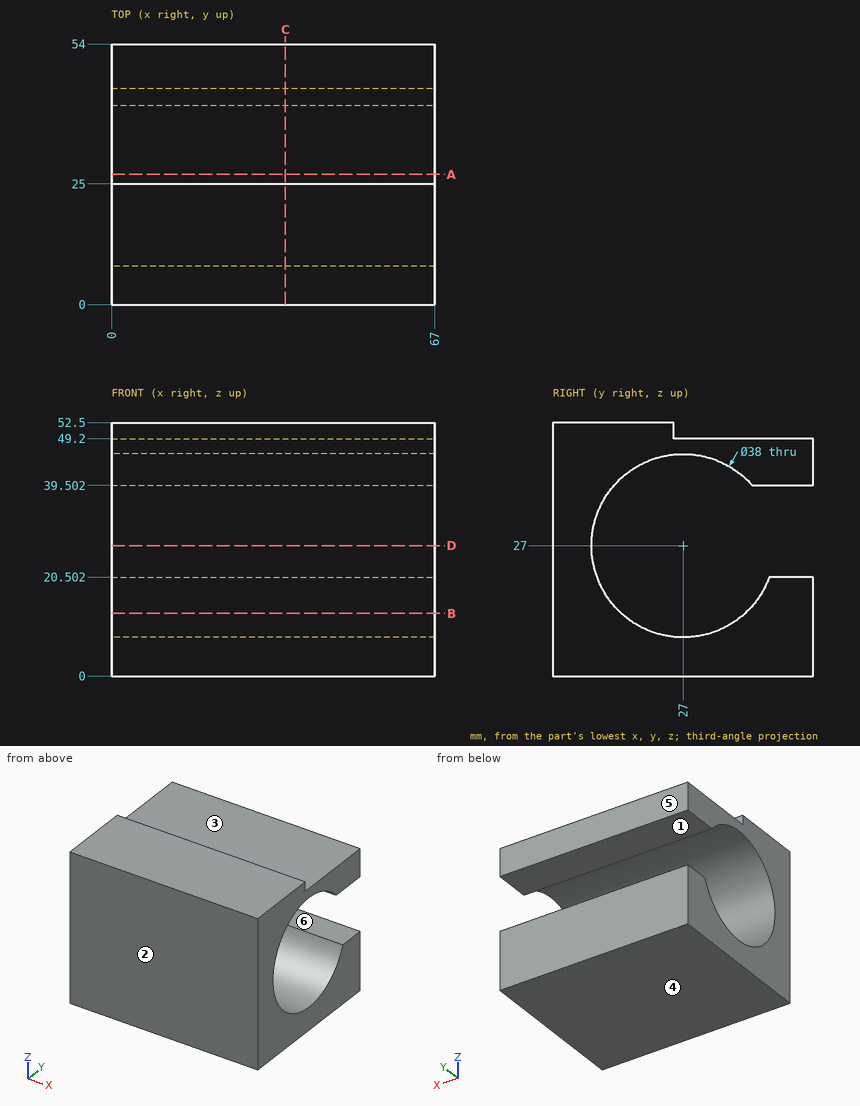
Check sheet for the drawn part. Datum: minimum x, y, z corner. Units: mm. A direction names the side the tool comes from. Round coordinates to 2 decimals unless told otherwise and drop trailing zeros. Order: outer loops, then holes, each group sorted by start corner. A loop starts at its lowest first (then second) coordinate and runs counter-clockwise, first axis right, second up. Notation, with made-up numbers: (86.25, 11) -> (142.25, 11) arc R18 cw to (142.25, 43) -> close; hole circle Ø2 at (-26.5, 70). An arc over 180 degrees is marked (long way). Put each result on its own line as item: value. Start each with the question number.
(1) Section check B-B (z = 13). Enter the section's corners in (x, y) (1 decimal), then the cut area to 3 significant figures.
(2) Depth check by flat-ended pin: pin 1 Ø2.5 at (x, z) = (44, 51) entering from +Y; pin 2 Ø12 at (x, y) = (55.5, 34.5) entering from -Z; pin 3 Ø4.5 at (x, y) = (50, 50) entering from +Z. Enter the tip coordinate at first touch or a pass-through.
(3) Section check D-D (z = 27). Enter the section's corners in (x, y).
(4) Draft check along Z on the marked faces 1, 2, 3 and 4. Enter one of: +Z half, -Z half, draft (parallel to the pull), parting line (faces both ways), or undercut.
(5) Tool access check on the marked faces 5 and 6. Record the directions out of +Z, -Z, +X, -X, +Y, -Y that give a thin tool (end or side, any length) a straight path to the whole face; none if there is none.
(6) Material ranges on line 1 along Z through (x, y) = (35, 49); line 2 along Y through (x, z) = (35, 27); line 3 along Z through (x, y) = (17.5, 27), recorded low to high.
(7) Section check C-C (x = 36). Enter the section's corners in (y, z), then the cut area to 3 significant figures.
(8) Section check A-A (y = 27). Enter the section's corners in (x, z).
Completed:
1. outline: (0, 0) -> (67, 0) -> (67, 14.2) -> (0, 14.2) -> close; (0, 39.8) -> (67, 39.8) -> (67, 54) -> (0, 54) -> close
1. area: 1,900 mm2
2. pin 1: stops at y = 25
2. pin 2: stops at z = 0
2. pin 3: stops at z = 49.2
3. outline: (0, 0) -> (67, 0) -> (67, 8) -> (0, 8) -> close
4. face 1: undercut
4. face 2: draft
4. face 3: +Z half
4. face 4: -Z half
5. face 5: +Z, -Z, +X, -X, +Y
5. face 6: +X, -X, +Y
6. line 1: z = 0 to 20.5, 39.5 to 49.2
6. line 2: y = 0 to 8
6. line 3: z = 0 to 8, 46 to 49.2
7. outline: (0, 0) -> (54, 0) -> (54, 20.5) -> (44.85, 20.5) arc R19 cw (long way) to (41.31, 39.5) -> (54, 39.5) -> (54, 49.2) -> (25, 49.2) -> (25, 52.5) -> (0, 52.5) -> close
7. area: 1,430 mm2
8. outline: (0, 0) -> (67, 0) -> (67, 8) -> (0, 8) -> close; (0, 46) -> (67, 46) -> (67, 49.2) -> (0, 49.2) -> close
